Answer from the drawing. Dimensions are ordinates in mm from the lowest x, y and z of the part. A direction names the side the tool comes from. Give positions to 0.01 mm unless a question says otherwise; leave off trailing zeros. Order: outer loops, then holes, each group sorted by start corner. A loop starts at its lowest first (then second) coordinate and runs counter-clockwise, first axis right, second up. Notation, with made-up numbers: (-1.5, 13) - (41.5, 13) arc R13 cw to (41.5, 22) - close; hole circle Ø11 at (56.5, 41). An arc over 180 degrees is marked (long way). One line per item, written item: value. Start each with the question number.
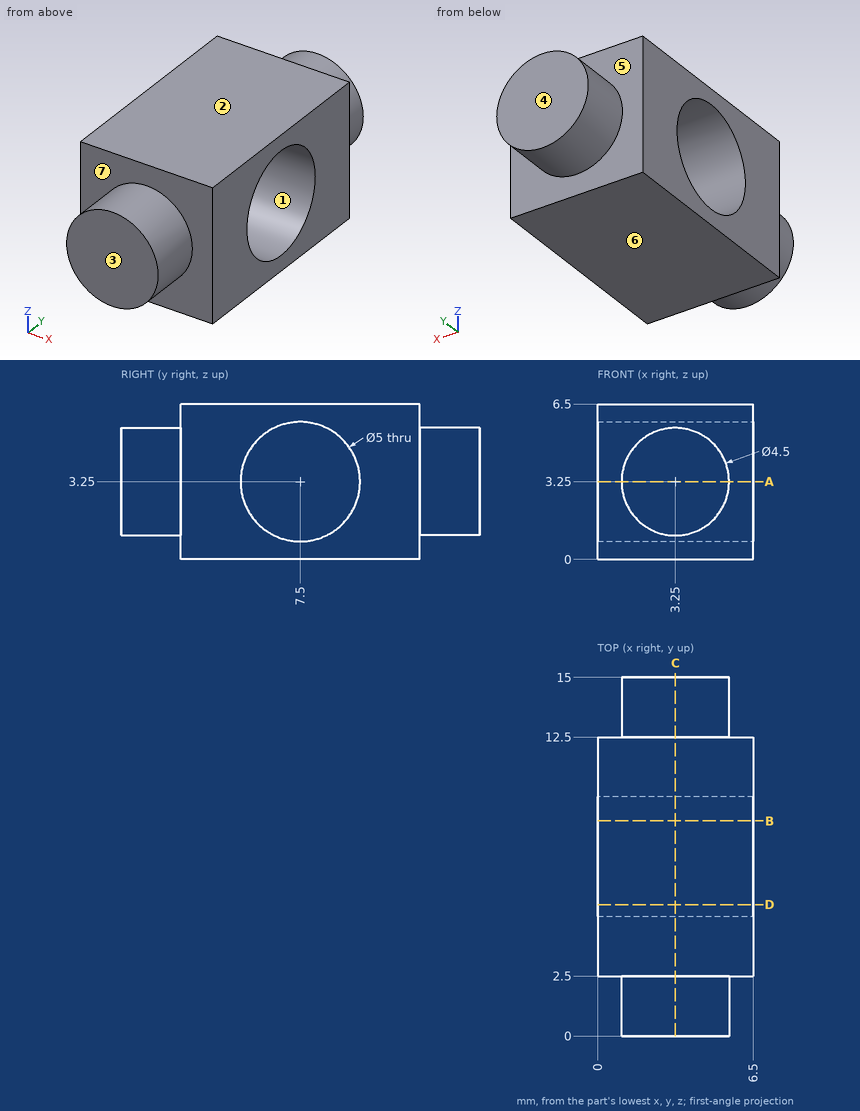
1) Find the intervals of material crossed by probe 1 along Z at (x, y) = (4, 7.5); probe 2 along Y at (x, z) = (3.5, 4.25); probe 3 along Y at (x, z) = (5.5, 2.75), in increasing order. Write a range as from..to.
2) Section B-B on y = 9 is taken. Write down the section's boundary in (x, z).
3) Section C-C on x = 3.25 is taken. Write down the section's boundary in (y, z).
4) Section A-A on z = 3.25 is taken. Write down the section's boundary in (x, y).
5) The mould has two halves that part along Y. Classify the marked faces 1, 2, 3 and 4: +Y half, -Y half, draft (parallel to the pull), parting line (faces both ways), or undercut.
6) Section D-D on y = 5.5 is taken. Write down the section's boundary in (x, z).
7) For the marked faces 5, 6 and 7, determine the directions among +Z, -Z, +X, -X, +Y, -Y from which every point of the face is accessible in a straight line to the end or side of a thin tool.
Solved:
1. probe 1: z = 0..0.75, 5.75..6.5
1. probe 2: y = 0..5.21, 9.79..15
1. probe 3: y = 2.5..5.05, 9.95..12.5
2. outline: (0, 0) - (6.5, 0) - (6.5, 1.25) - (0, 1.25) - close; (0, 5.25) - (6.5, 5.25) - (6.5, 6.5) - (0, 6.5) - close
3. outline: (0, 1) - (2.5, 1) - (2.5, 0) - (12.5, 0) - (12.5, 1) - (15, 1) - (15, 5.5) - (12.5, 5.5) - (12.5, 6.5) - (2.5, 6.5) - (2.5, 5.5) - (0, 5.5) - close; hole circle Ø5 at (7.5, 3.25)
4. outline: (0, 2.5) - (1, 2.5) - (1, 0) - (5.5, 0) - (5.5, 2.5) - (6.5, 2.5) - (6.5, 5) - (0, 5) - close; (0, 10) - (6.5, 10) - (6.5, 12.5) - (5.5, 12.5) - (5.5, 15) - (1, 15) - (1, 12.5) - (0, 12.5) - close
5. face 1: undercut
5. face 2: draft
5. face 3: -Y half
5. face 4: +Y half
6. outline: (0, 0) - (6.5, 0) - (6.5, 1.75) - (0, 1.75) - close; (0, 4.75) - (6.5, 4.75) - (6.5, 6.5) - (0, 6.5) - close
7. face 5: +Y
7. face 6: -Z, +X, -X, +Y, -Y
7. face 7: -Y
